```python
from build123d import *

# Parameters (mm, degrees)
SKETCH_W     = 605
SKETCH_H     = 605
PAD_DEPTH    = 18
SKETCH001_R  = 3.175
PAD001_DEPTH = 20
SKETCH002_R  = 3.175
POCKET_DEPTH = 3


with BuildPart() as part:
    # Sketch → Pad (new body)
    with BuildSketch(Plane.XY):
        Rectangle(SKETCH_W, SKETCH_H)
    extrude(amount=PAD_DEPTH)

    # Sketch001 (on Face6 of Pad) → Pad001 (join)
    with BuildSketch(Plane.XY.offset(18)):
        with Locations((-100, 0)):
            Circle(SKETCH001_R)
        with Locations((100, 0)):
            Circle(SKETCH001_R)
    extrude(amount=PAD001_DEPTH)

    # Sketch002 (on Face5 of Pad001) → Pocket (cut)
    with BuildSketch(Plane.XY.offset(18)):
        with Locations((-200, 0)):
            Circle(SKETCH002_R)
        Circle(SKETCH002_R)
        with Locations((200, 0)):
            Circle(SKETCH002_R)
    extrude(amount=-POCKET_DEPTH, mode=Mode.SUBTRACT)


solid = part.part
```
Work out the finished part from the listing and answer in its coordinate system (mm). Round coordinates to 2 decimals unless told otherwise and drop trailing zeros. Loops run counter-clockwise (first coordinate to the right, second up) from the corner with the lowest first, then second, coordinate; pieces in that order, holes last. Notation, with made-up numbers: (4.5, -9) -> (60.5, -9) arc R20 cw to (60.5, 20) -> close; hole circle Ø8 at (-1.5, 16). An arc over 180 degrees is marked (long way). Write each question's results on one line, items separated by ' | '. Start each with the question number.
1. For a pull along X with two mould halves and no side action, classify faces 1 (the face through (-4, 4, 0)), 2 (the face through (302.5, -4, 9)), 3 (the face through (-302.5, -4, 9)) as +X half, -X half, draft (parallel to the pull), parting line (faces both ways), or undercut.
2. Find the intervals of material crossed by probe 1 along Y at (x, z) = (0, 15.8) (3 decimals); probe 2 along Z at (x, y) = (-276, -206); probe 3 along X at (y, z) = (2, 25.5), in increasing order. Write a range as from..to.
3. Given pin 1 Ø4 at (x, y) = (200, 0) entering from +Z; pin 2 Ø7 at (x, y) = (-200.5, -1.5) entering from +Z, each flat-ended and moving along its own axis, determine where each tip first touches the part or whether it passes through.
4. Section A-A (y = -181) is taken. Determine the outline of the cut face in (x, z).
Evaluation:
1) face 1: draft | face 2: +X half | face 3: -X half
2) probe 1: y = -302.5..-3.175, 3.175..302.5 | probe 2: z = 0..18 | probe 3: x = -102.47..-97.53, 97.53..102.47
3) pin 1: stops at z = 15 | pin 2: stops at z = 18
4) outline: (-302.5, 0) -> (302.5, 0) -> (302.5, 18) -> (-302.5, 18) -> close
